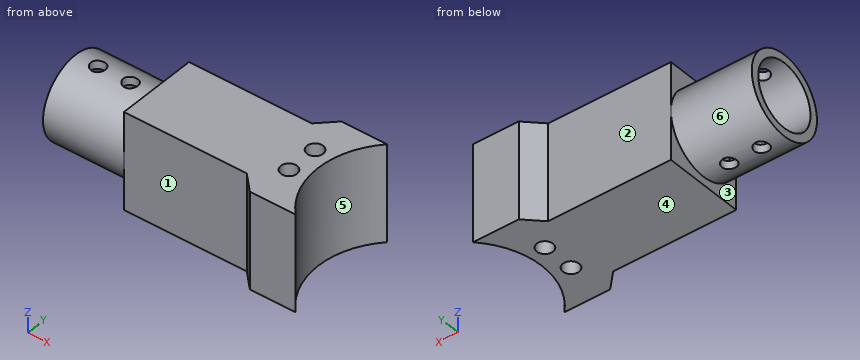
Solid Edge part; units mm, degrees
sketch "Sketch1" plane through (0, 0, 0) normal (0, 0, 1) x (1, 0, 0)
  line L0 (-25, -12.5) -> (25, -12.5)
  line L1 (25, -12.5) -> (25, 12.5)
  line L2 (25, 12.5) -> (-25, 12.5)
  line L3 (-25, 12.5) -> (-25, -12.5)
  circle A0 centre (20, 5) radius 2.5
  circle A1 centre (20, -5) radius 2.5
extrude "Protrusion1" add sketch "Sketch1" along normal mid plane 30
sketch "Sketch2" plane through (-25, 0, 0) normal (-1, 0, 0) x (0, -1, 0)
  circle A0 centre (0, 0) radius 10
  circle A1 centre (0, 0) radius 12.5
extrude "ExtrudedProtrusion_2" add sketch "Sketch2" along normal mid plane 50
sketch "Sketch3" plane through (0, 0, 0) normal (0, 0, 1) x (1, 0, 0)
  arc A0 (32.1464, 17.5) -> (32.1464, -17.5) centre (50, 0) ccw
  line L0 (32.1464, -17.5) -> (18, -17.5)
  line L1 (18, -17.5) -> (13, -12.5)
  line L2 (13, -12.5) -> (22.5, -12.5)
  line L3 (22.5, -12.5) -> (22.5, 12.5)
  line L4 (22.5, 12.5) -> (13, 12.5)
  line L5 (13, 12.5) -> (18, 17.5)
  line L6 (18, 17.5) -> (32.1464, 17.5)
extrude "Protrusion2" add sketch "Sketch3" along normal mid plane 30
sketch "Sketch4" plane through (0, 0, 0) normal (0, 0, 1) x (1, 0, 0)
  circle A0 centre (-43, 0) radius 2.25
  circle A1 centre (-33, 0) radius 2.25
extrude "ExtrudedCutout_1" cut sketch "Sketch4" along normal mid plane 87.851
properties material "PVC"
For this review, take the finished solid that the model builds, in its own axes (mm). Face numbers are marked on the shaded views. A direction names the side the tool comes from. Coordinates: 2 decimals unless noted, no trailing zeros. Write each loop counter-clockwise with the first axis right and the second up, starting at its lowest first coordinate (ties: lowest second). Pieces come first, ordered by that corner, then holes.
(1) Add section B-B on x = 20. Give the boundary of the cut face in (y, z).
(2) The part is to be moulded in two halves that separate along Y. For the marked faces 4, 5 and 6, say which applies: +Y half, -Y half, draft (parallel to the pull), parting line (faces both ways), or undercut.
(3) Tool access review of the marked faces 1, 2 and 3: name each direction out of +Z, -Z, +X, -X, +Y, -Y from which nothing blocks a thin tool from reaching the whole face with its end or side.
(4) Add section D-D on z = 6.25. Give the boundary of the cut face in (x, y).
(5) For pin 1 Ø12 at (x, z) = (-40.5, 3) entering from +Y; pin 2 Ø12 at (y, z) = (0, 0) entering from +X; pin 3 Ø5 at (x, y) = (-33, 0) entering from +Z; pin 4 Ø3.5 at (x, y) = (-43, 0) entering from -Z, all flat-tipped, find the tip position at first contact; note any pin that passes through.
(6) Add section A-A on y = 0. Give the boundary of the cut face in (x, z), then the cut area to 3 significant figures.
(7) Add section C-C on z = -4.25. Give the boundary of the cut face in (x, y), then the cut area to 3 significant figures.
(8) Wall thickness on probe 1 along X at (y, z) = (0, -10.8); probe 2 along Y at (x, z) = (20, -5.25); probe 3 along Y at (x, z) = (18, 12): over which ranges is each line inside the solid? List them lowest first.
Answer sheet:
1. outline: (-17.5, -15) - (-7.5, -15) - (-7.5, 15) - (-17.5, 15) - close; (-2.5, -15) - (2.5, -15) - (2.5, 15) - (-2.5, 15) - close; (7.5, -15) - (17.5, -15) - (17.5, 15) - (7.5, 15) - close
2. face 4: draft
2. face 5: undercut
2. face 6: parting line
3. face 1: +Z, -Z, -X, -Y
3. face 2: +Z, -Z, -X, +Y
3. face 3: -Z, -X
4. outline: (-50, -10.83) - (-25, -10.83) - (-25, -12.5) - (13, -12.5) - (18, -17.5) - (32.15, -17.5) arc R25 cw to (32.15, 17.5) - (18, 17.5) - (13, 12.5) - (-25, 12.5) - (-25, 10.83) - (-50, 10.83) - (-50, 7.81) - (-25, 7.81) - (-25, -7.81) - (-50, -7.81) - close; hole circle Ø5 at (20, -5); hole circle Ø5 at (20, 5)
5. pin 1: stops at y = 12.5
5. pin 2: stops at x = 25.73
5. pin 3: stops at z = 12.5
5. pin 4: passes through
6. outline: (-50, -12.5) - (-45.25, -12.5) - (-45.25, -10) - (-50, -10) - close; (-50, 10) - (-45.25, 10) - (-45.25, 12.5) - (-50, 12.5) - close; (-40.75, -12.5) - (-35.25, -12.5) - (-35.25, -10) - (-40.75, -10) - close; (-40.75, 10) - (-35.25, 10) - (-35.25, 12.5) - (-40.75, 12.5) - close; (-30.75, -12.5) - (-25, -12.5) - (-25, -15) - (25, -15) - (25, 15) - (-25, 15) - (-25, 12.5) - (-30.75, 12.5) - (-30.75, 10) - (-25, 10) - (-25, -10) - (-30.75, -10) - close
6. area: 1,580 mm2
7. outline: (-50, -11.76) - (-25, -11.76) - (-25, -12.5) - (13, -12.5) - (18, -17.5) - (32.15, -17.5) arc R25 cw to (32.15, 17.5) - (18, 17.5) - (13, 12.5) - (-25, 12.5) - (-25, 11.76) - (-50, 11.76) - (-50, 9.05) - (-25, 9.05) - (-25, -9.05) - (-50, -9.05) - close; hole circle Ø5 at (20, -5); hole circle Ø5 at (20, 5)
7. area: 1,520 mm2
8. probe 1: x = -50 to -45.25, -40.75 to -35.25, -30.75 to 25
8. probe 2: y = -17.5 to -7.5, -2.5 to 2.5, 7.5 to 17.5
8. probe 3: y = -17.5 to -6.5, -3.5 to 3.5, 6.5 to 17.5
